Study the drawing (mm; zero at the part's minimum x, y, z) and answer. Round coordinates to 2 decimals unless told otherwise and drop trailing zeros. Order: outer loops, then holes, each group sorted by start corner. A loop starts at its lowest first (then second) coordinate and runs counter-clockwise, first axis right, second up. Notation, with made-up numbers: (43, 52) - (78, 52) arc R20 cw to (78, 87) - close; hole circle Ø1 at (13.25, -5). An arc over 180 degrees is marked (long way). Use one line per item in the form item = value. Start each with the question number.
Q1. The part is cut by section C-C on y = 2. Determine the outline of the cut face in (x, z).
Q2. Find the intervals of material crossed by line 1 (Y direction, x = 5, z = 9.75); line 2 (X direction, y = 4.5, z = 4.25) (1 decimal); line 3 (Y direction, x = 6.5, z = 2.5), in increasing order. Write a range as [from, to].
Q3. Given P1, Ø2, axis at x = 5, y = 4.5, coming from the -Z side; P2, Ø1.5, axis at x = 8.5, z = 10, coming from the -Y side; P3, Ø4, axis at x = 2, z = 4.5, coming from the -Y side, each flat-ended and moving along its own axis, determine where each tip first touches the part or whether it passes through.
Q4. The part is cut by section D-D on x = 9.25. Determine the outline of the cut face in (y, z).
Q5. The part is cut by section B-B on z = 8.75. Determine the outline of the cut face in (x, y).
Q6. For a pull along X with two mould halves and no side action, classify the marked faces 1, 2, 3 and 4 as +X half, -X half, draft (parallel to the pull), parting line (faces both ways), or undercut.
Q7. The part is cut by section A-A on x = 5. Determine the outline of the cut face in (y, z) (3 decimals), plus the area to 3 significant figures.
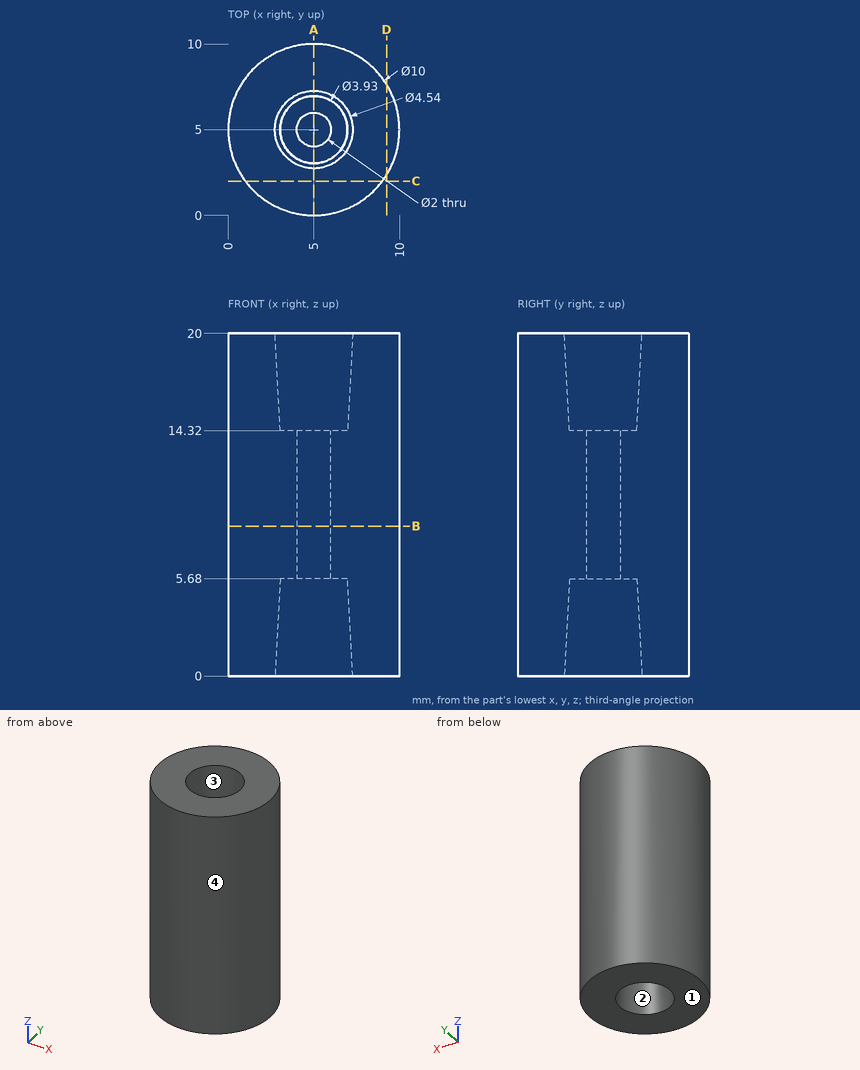
Found:
q1.outline = (1, 0) - (9, 0) - (9, 20) - (1, 20) - close
q2.line_1 = [0, 4], [6, 10]
q2.line_2 = [0, 3], [7, 10]
q2.line_3 = [0.23, 3.48], [6.52, 9.77]
q3.P1 = 5.68
q3.P2 = 0.82
q3.P3 = 0.1
q4.outline = (2.37, 0) - (7.63, 0) - (7.63, 20) - (2.37, 20) - close
q5.outline = circle Ø10 at (5, 5); hole circle Ø2 at (5, 5)
q6.face_1 = draft
q6.face_2 = undercut
q6.face_3 = undercut
q6.face_4 = parting line
q7.outline = (0, 0) - (2.73, 0) - (3.035, 5.68) - (4, 5.68) - (4, 14.32) - (3.035, 14.32) - (2.73, 20) - (0, 20) - close; (6, 5.68) - (6.965, 5.68) - (7.27, 0) - (10, 0) - (10, 20) - (7.27, 20) - (6.965, 14.32) - (6, 14.32) - close
q7.area = 135 mm²
